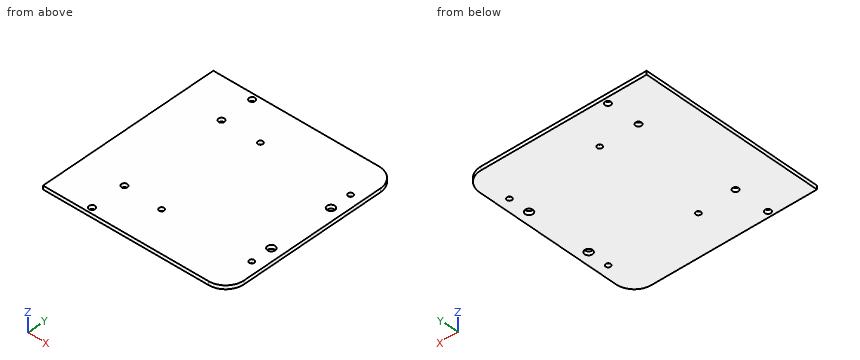
from build123d import *

# Parameters (mm, degrees)
EXTRUDE_1_DEPTH     = 2
SKETCH_3_R          = 1.35
CUT_EXTRUDE_1_DEPTH = 3
SKETCH_7_R          = 2.1
CUT_EXTRUDE_5_DEPTH = 10
SKETCH_8_R          = 1.6
CUT_EXTRUDE_6_DEPTH = 3


with BuildPart() as part:
    # 草图1 → 凸台-拉伸1 (new body)
    with BuildSketch(Plane.XY):
        with BuildLine():
            Line((-50, 50), (40, 50))
            ThreePointArc((40, 50), (47.071067812, 47.071067812), (50, 40))
            Line((50, 40), (50, -40))
            ThreePointArc((50, -40), (47.071067812, -47.071067812), (40, -50))
            Line((40, -50), (-50, -50))
            Line((-50, -50), (-50, 50))
        make_face()
    extrude(amount=EXTRUDE_1_DEPTH)

    # 草图3 → 切除-拉伸1 (cut, through all)
    with BuildSketch(Plane.XY.offset(2)):
        with Locations((-5, -29)):
            Circle(SKETCH_3_R)
        with Locations((-5, 29)):
            Circle(SKETCH_3_R)
        with Locations((44, 29)):
            Circle(SKETCH_3_R)
        with Locations((44, -29)):
            Circle(SKETCH_3_R)
    extrude(amount=-CUT_EXTRUDE_1_DEPTH, mode=Mode.SUBTRACT)

    # 草图7 → 切除-拉伸5 (cut)
    with BuildSketch(Plane.XY.offset(2)):
        with Locations((44, 17.5)):
            Circle(SKETCH_7_R)
        with Locations((44, -17.5)):
            Circle(SKETCH_7_R)
    extrude(amount=-CUT_EXTRUDE_5_DEPTH, mode=Mode.SUBTRACT)

    # 草图8 → 切除-拉伸6 (cut, through all)
    with BuildSketch(Plane(origin=(0, 0, 0), x_dir=(-1, 0, 0), z_dir=(0, 0, -1))):
        with Locations((26.125, -47)):
            Circle(SKETCH_8_R)
        with Locations((26.125, -28)):
            Circle(SKETCH_8_R)
        with Locations((26.125, 29)):
            Circle(SKETCH_8_R)
        with Locations((26.125, 47)):
            Circle(SKETCH_8_R)
    extrude(amount=-CUT_EXTRUDE_6_DEPTH, mode=Mode.SUBTRACT)


solid = part.part
Work out the finished part from the listing and answer in its coordinate system (mm). Round coordinates to 2 decimals unless told otherwise and drop trailing zeros. Write each loop counter-clockwise with the first axis right and the second up, starting at its lowest first coordinate (ties: lowest second). Pieces come first, ordered by that corner, then holes. Notation, with made-up numbers: (-15.75, 2.5) - (38.25, 2.5) arc R20 cw to (38.25, 14.5) - close; hole circle Ø4 at (64.25, 89). An arc over 180 degrees is marked (long way). Answer in a Markdown table with one row per item. Add a question column.
1. A cutting plane is placed at D-D, the plane x = 44. Determine the outline of the cut face in (y, z).
2. A cutting plane is placed at B-B, the plane x = -5. Determine the outline of the cut face in (y, z), and give its area (3 significant figures).
3. Find the intervals of material crossed by line 1 along Y through (x, z) = (44, 1.2); line 2 along X through (y, z) = (-17, 1.9); line 3 along X through (y, z) = (-43, 0.3), in increasing order. Write a range as from..to.
4. A cutting plane is placed at A-A, the plane y = 29. Determine the outline of the cut face in (x, z) (3 decimals).
5. Given pin 1 (4 mm diameter, centred on x = 44, y = -17.5, fed in from -Z), flat-ended and moving along its own axis, determine where the tip first touches the part or whether it passes through.
6. A cutting plane is placed at C-C, the plane y = 17.5. Determine the outline of the cut face in (x, z), and give its area (3 significant figures).
Worked out:
| question | item | result |
|---|---|---|
| 1 | outline | (-49.17, 0) - (-30.35, 0) - (-30.35, 2) - (-49.17, 2) - close; (-27.65, 0) - (-19.6, 0) - (-19.6, 2) - (-27.65, 2) - close; (-15.4, 0) - (15.4, 0) - (15.4, 2) - (-15.4, 2) - close; (19.6, 0) - (27.65, 0) - (27.65, 2) - (19.6, 2) - close; (30.35, 0) - (49.17, 0) - (49.17, 2) - (30.35, 2) - close |
| 2 | outline | (-50, 0) - (-30.35, 0) - (-30.35, 2) - (-50, 2) - close; (-27.65, 0) - (27.65, 0) - (27.65, 2) - (-27.65, 2) - close; (30.35, 0) - (50, 0) - (50, 2) - (30.35, 2) - close |
| 2 | area | 189 mm^2 |
| 3 | line 1 | -49.17..-30.35, -27.65..-19.6, -15.4..15.4, 19.6..27.65, 30.35..49.17 |
| 3 | line 2 | -50..41.96, 46.04..50 |
| 3 | line 3 | -50..49.54 |
| 4 | outline | (-50, 0) - (-27.725, 0) - (-27.725, 2) - (-50, 2) - close; (-24.525, 0) - (-6.35, 0) - (-6.35, 2) - (-24.525, 2) - close; (-3.65, 0) - (42.65, 0) - (42.65, 2) - (-3.65, 2) - close; (45.35, 0) - (50, 0) - (50, 2) - (45.35, 2) - close |
| 5 | pin 1 | through |
| 6 | outline | (-50, 0) - (41.9, 0) - (41.9, 2) - (-50, 2) - close; (46.1, 0) - (50, 0) - (50, 2) - (46.1, 2) - close |
| 6 | area | 192 mm^2 |
